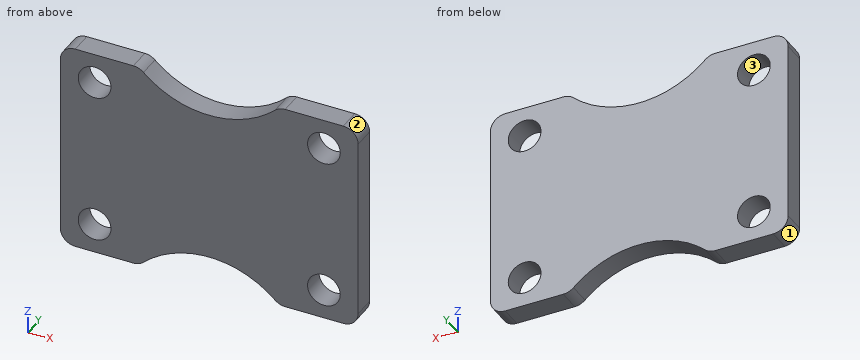
from build123d import *

# Parameters (mm, degrees)
F0_W     = 20
F0_H     = 14.2
F1_DEPTH = 1.5
F2_R     = 1.1
F3_DEPTH = 1.5
F4_R     = 1


with BuildPart() as f1:
    # F0 (on Front) → F1 (new body)
    with BuildSketch(Plane.XZ):
        with Locations((10, 7.1)):
            Rectangle(F0_W, F0_H)
    extrude(amount=F1_DEPTH)

    # F2 (on face) → F3 (cut, through all)
    with BuildSketch(Plane.XZ.offset(1.5)):
        with Locations((2.3, 12.2)):
            Circle(F2_R)
        with Locations((17.7, 12.2)):
            Circle(F2_R)
        with Locations((2.3, 2)):
            Circle(F2_R)
        with Locations((17.7, 2)):
            Circle(F2_R)
        with BuildLine():
            Line((14.6904157598, 14.2), (5.3095842402, 14.2))
            ThreePointArc((5.3095842402, 14.2), (10, 12.2), (14.6904157598, 14.2))
        make_face()
        with BuildLine():
            ThreePointArc((14.6904157598, 0), (10, 2), (5.3095842402, 0))
            Line((5.3095842402, 0), (14.6904157598, 0))
        make_face()
    extrude(amount=-F3_DEPTH, mode=Mode.SUBTRACT)

    # F4
    f4_edges = [f1.edges().sort_by_distance(p)[0] for p in [
        (20, -0.75, 14.2),
        (20, -0.75, 0),
        (0, -0.75, 14.2),
        (0, -0.75, 0),
        (5.309584, -0.75, 14.2),
        (14.690416, -0.75, 14.2),
        (5.309584, -0.75, 0),
        (14.690416, -0.75, 0),
    ]]
    fillet(f4_edges, radius=F4_R)


solid = f1.part
Source: CAD feature listing. Evaluate the final solid. Frame: model axes, mm. Face numbers are marked on the shaded views. Give positions to 0.01 mm unless a question says otherwise; leave off trailing zeros. Write each loop counter-clockwise with the first axis right and the second up, starting at its lowest first coordinate (ties: lowest second). Pieces come first, ordered by that corner, then holes. Notation, with made-up numbers: (8, 22) -> (15, 22) arc R24 ccw to (15, 61) -> close; hole circle Ø9 at (-20, 38.25). An arc over 180 degrees is marked (long way). Write item = value, one per line.
Q1. Cut plane C-C on z = 12. Return loops of the section in (x, y).
Here are the results:
outline = (0, -1.5) -> (1.22, -1.5) -> (1.22, 0) -> (0, 0) -> close; (3.38, -1.5) -> (16.62, -1.5) -> (16.62, 0) -> (3.38, 0) -> close; (18.78, -1.5) -> (20, -1.5) -> (20, 0) -> (18.78, 0) -> close
Q2. Mould query, pull axis X, two halves, no side actions, for the marked faces 1, 2 and 3. Classes: +X half, -X half, draft (parallel to the pull), parting line (faces both ways), or undercut.
Here are the results:
face_1 = -X half
face_2 = +X half
face_3 = undercut
Q3. Cut plane D-D on x = 8. Return loops of the section in (y, z).
Here are the results:
outline = (-1.5, 1.68) -> (0, 1.68) -> (0, 12.52) -> (-1.5, 12.52) -> close
Q4. Cut plane A-A on y = -0.95. Return loops of the section in (x, z), then the cut area to 3 significant figures.
Here are the results:
outline = (0, 1) arc R1 ccw to (1, 0) -> (4.9, 0) arc R1 ccw to (5.58, 0.27) arc R6.5 cw to (14.42, 0.27) arc R1 ccw to (15.1, 0) -> (19, 0) arc R1 ccw to (20, 1) -> (20, 13.2) arc R1 ccw to (19, 14.2) -> (15.1, 14.2) arc R1 ccw to (14.42, 13.93) arc R6.5 cw to (5.58, 13.93) arc R1 ccw to (4.9, 14.2) -> (1, 14.2) arc R1 ccw to (0, 13.2) -> close; hole circle Ø2.2 at (2.3, 2); hole circle Ø2.2 at (2.3, 12.2); hole circle Ø2.2 at (17.7, 2); hole circle Ø2.2 at (17.7, 12.2)
area = 242 mm²
Q5. Line query: line 1 (Z direction, x = 17.7, y = -0.5); line 2 (X direction, y = -0.6, z = 11.5); line 3 (Z direction, x = 2.75, y = -1.1). Output: solid intervals per line, ascending. Write a range as from..to.
Here are the results:
line_1 = 0..0.9, 3.1..11.1, 13.3..14.2
line_2 = 0..1.45, 3.15..16.85, 18.55..20
line_3 = 0..1, 3..11.2, 13.2..14.2
Q6. Cut plane B-B on x = 17.7. Return loops of the section in (y, z).
Here are the results:
outline = (-1.5, 0) -> (0, 0) -> (0, 0.9) -> (-1.5, 0.9) -> close; (-1.5, 3.1) -> (0, 3.1) -> (0, 11.1) -> (-1.5, 11.1) -> close; (-1.5, 13.3) -> (0, 13.3) -> (0, 14.2) -> (-1.5, 14.2) -> close
